Geometry: final body of the model. Coordinates: model frame, mm. Face numbers are marked on the shaded views. A direction names the side the tool comes from. Coordinates: 2 decimals unless noted, no trailing zeros. Write each loop counter-clockwise with the first axis right and the second up, starting at its lowest first coordinate (ties: lowest second). Pieces come first, ordered by that corner, then holes. Notation, with made-up numbers: (13, 46.25) - (71, 46.25) arc R12 ccw to (71, 67.25) - close; hole circle Ø5 at (-27.75, 48). An arc over 180 degrees is marked (long way). Answer as a JSON object with one key per item and string values. Group by question number.
Item 1: Section A-A on x = 2. Return loops of the section in (y, z), and give its area (3 significant figures).
Item 2: Set-up query: the marked faces 1, 2 and 3. Return all of +Z, -Z, +X, -X, +Y, -Y with unobstructed straight access to the full face (end or side cutting, diameter ignored); none if empty.
Item 3: Section D-D on z = 9. Return loops of the section in (x, y).
Item 4: Mould query, pull axis Z, two halves, no side actions, for the marked faces 4, 5 and 6. Classes: pulls with the +Z half, pulls with the -Z half, needs draft (parallel to the pull), parting line crosses it, or undercut.
Item 5: Section C-C on y = 8. Return loops of the section in (x, z).
Item 6: Line query: line 1 along Z through (x, y) = (0.4, 3); line 2 along Z through (x, y) = (2.1, 1); line 3 along Z through (x, y) = (4.4, 4). Output: solid intervals per line, ascending. Write a range as from..to.
Item 7: First-contact query: pin 1 Ø0.8 at (x, y) = (2.5, 9) entering from -Z; pin 2 Ø1 at (x, y) = (3, -7.5) entering from +Z; pin 3 Ø2.5 at (x, z) = (2, 3.5) entering from -Y. Flat tips, straight axial feed; report the tip coordinate or a pass-through.
Item 8: Section B-B on z = -4. Return loops of the section in (x, y), and give its area (3 significant figures).
```python
from build123d import *

# Parameters (mm, degrees)
SKETCH1_R           = 1.2295
SKETCH1_R_2         = 2
SKETCH1_R_3         = 1
BOSS_EXTRUDE1_DEPTH = 5
SKETCH2_R           = 1.25
CUT_EXTRUDE1_DEPTH  = 5
FILLET1_R           = 5


with BuildPart() as part:
    # Sketch1 → Boss-Extrude1 (new body)
    with BuildSketch(Plane.YZ):
        with BuildLine():
            Line((-11.729138766, -13.432284692), (-11.729138766, -7.362284692))
            ThreePointArc((-11.729138766, -7.362284692), (-10.85045911, -5.240964348), (-8.729138766, -4.362284692))
            Line((-8.729138766, -4.362284692), (-6.729138766, -4.362284692))
            ThreePointArc((-6.729138766, -4.362284692), (-4.607818422, -3.483605035), (-3.729138766, -1.362284692))
            Line((-3.729138766, -1.362284692), (-3.729138766, 11.567715308))
            Line((-3.729138766, 11.567715308), (9.270861234, 11.567715308))
            Line((9.270861234, 11.567715308), (9.270861234, 8.567715308))
            Line((9.270861234, 8.567715308), (9.270861234, -3.189644004))
            ThreePointArc((9.270861234, -3.189644004), (9.499222636, -4.337694301), (10.14954089, -5.310964348))
            Line((10.14954089, -5.310964348), (11.392181578, -6.553605035))
            ThreePointArc((11.392181578, -6.553605035), (12.042499832, -7.526875082), (12.270861234, -8.674925379))
            Line((12.270861234, -8.674925379), (12.270861234, -13.432284692))
            Line((12.270861234, -13.432284692), (-11.729138766, -13.432284692))
        make_face()
        with Locations(Location((3.770861234, 5.137715308, 0), (0, 0, 270))):
            Circle(SKETCH1_R, mode=Mode.SUBTRACT)
        with Locations(Location((2.770861234, -0.362284692, 0), (0, 0, 270))):
            Circle(SKETCH1_R_2, mode=Mode.SUBTRACT)
        with Locations(Location((3.770861234, -4.362284692, 0), (0, 0, 270))):
            Circle(SKETCH1_R, mode=Mode.SUBTRACT)
        with Locations(Location((-8.729138766, -7.362284692, 0), (0, 0, 270))):
            Circle(SKETCH1_R, mode=Mode.SUBTRACT)
        with Locations(Location((-8.729138766, -10.932284692, 0), (0, 0, 270))):
            Circle(SKETCH1_R_3, mode=Mode.SUBTRACT)
        with Locations(Location((1.270861234, -10.932284692, 0), (0, 0, 270))):
            Circle(SKETCH1_R_3, mode=Mode.SUBTRACT)
    extrude(amount=BOSS_EXTRUDE1_DEPTH)

    # Sketch2 → Cut-Extrude1 (cut)
    with BuildSketch(Plane(origin=(0, 0, -13.432284692), x_dir=(1, 0, 0), z_dir=(0, 0, -1))):
        with Locations(Location((2.5, -8.770861234, 0), (0, 0, 180))):
            Circle(SKETCH2_R)
        with Locations(Location((2.5, 5.229138766, 0), (0, 0, 180))):
            Circle(SKETCH2_R)
    extrude(amount=-CUT_EXTRUDE1_DEPTH, mode=Mode.SUBTRACT)

    # Fillet1
    fillet1_edges = [part.edges().sort_by_distance(p)[0] for p in [
        (2.5, -3.729138766, 11.567715308),
        (2.5, 9.270861234, 11.567715308),
    ]]
    fillet(fillet1_edges, radius=FILLET1_R)


solid = part.part
```
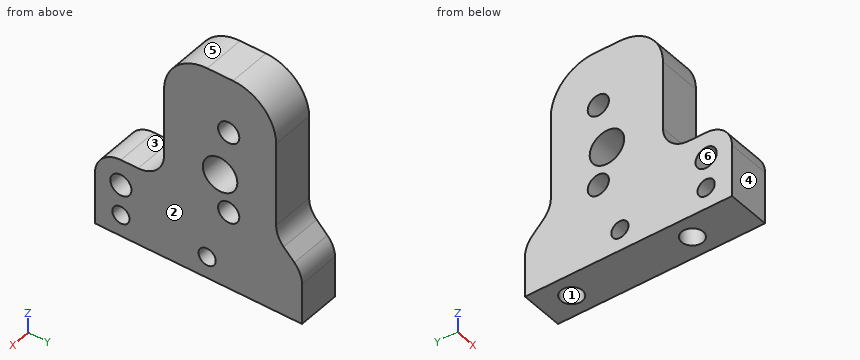
Checks:
{
 "1": {"outline": "(-11.73, -13.43) - (-6.37, -13.43) - (-6.37, -8.43) - (-4.08, -8.43) - (-4.08, -13.43) - (7.63, -13.43) - (7.63, -8.43) - (9.92, -8.43) - (9.92, -13.43) - (12.27, -13.43) - (12.27, -8.67) arc R3 ccw to (11.39, -6.55) - (10.15, -5.31) arc R3 cw to (9.27, -3.19) - (9.27, 6.57) arc R5 ccw to (4.27, 11.57) - (1.27, 11.57) arc R5 ccw to (-3.73, 6.57) - (-3.73, -1.36) arc R3 cw to (-6.73, -4.36) - (-8.73, -4.36) arc R3 ccw to (-11.73, -7.36) - close; hole circle Ø2.46 at (-8.73, -7.36); hole circle Ø2 at (-8.73, -10.93); hole circle Ø2 at (1.27, -10.93); hole circle Ø4 at (2.77, -0.36); hole circle Ø2.46 at (3.77, -4.36); hole circle Ø2.46 at (3.77, 5.14)", "area": "353 mm^2"},
 "2": {"face 1": "-Z", "face 2": "+Z, -Z, +X, +Y, -Y", "face 3": "+Z, +X, -X, -Y"},
 "3": {"outline": "(0, -3.1) - (5, -3.1) - (5, 8.64) - (0, 8.64) - close"},
 "4": {"face 4": "needs draft", "face 5": "pulls with the +Z half", "face 6": "undercut"},
 "5": {"outline": "(0, -13.43) - (1.52, -13.43) - (1.52, -8.43) - (3.48, -8.43) - (3.48, -13.43) - (5, -13.43) - (5, 9.9) - (0, 9.9) - close"},
 "6": {"line 1": "-13.43..-5.32, -3.4..-2.35, 1.62..4.18, 6.1..11.57", "line 2": "-13.43..-11.89, -9.97..-1.29, 0.57..11.56", "line 3": "-13.43..-5.57, -3.15..-1.94, 1.22..3.93, 6.35..11.57"},
 "7": {"pin 1": "z = -8.43", "pin 2": "z = -4.36", "pin 3": "y = -3.73"},
 "8": {"outline": "(0, -5.3) - (5, -5.3) - (5, 2.6) - (0, 2.6) - close; (0, 4.95) - (5, 4.95) - (5, 9.38) - (0, 9.38) - close", "area": "61.7 mm^2"}
}
